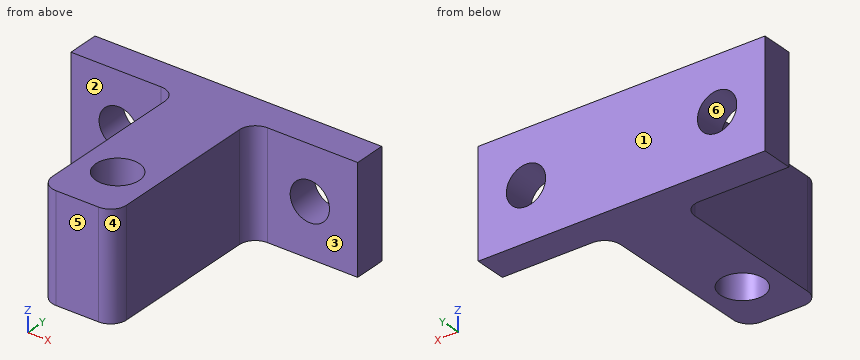
from build123d import *

# Parameters (mm, degrees)
SKETCH1_R           = 2.05
BOSS_EXTRUDE1_DEPTH = 5
FILLET1_R           = 1.5
SKETCH2_R           = 1.85
CUT_EXTRUDE1_DEPTH  = 21


with BuildPart() as part:
    # Sketch1 → Boss-Extrude1 (new body, symmetric)
    with BuildSketch(Plane.XY):
        Polygon((-13.502392344, 0), (-3.5, 0), (-3.5, -17), (3.5, -17), (3.5, 0), (13.502392344, 0), (13.502392344, 3), (-13.502392344, 3), align=None)
        with Locations((0, -12)):
            Circle(SKETCH1_R, mode=Mode.SUBTRACT)
    extrude(amount=BOSS_EXTRUDE1_DEPTH, both=True)

    # Fillet1
    fillet1_edges = [part.edges().sort_by_distance(p)[0] for p in [
        (3.5, 0, 0),
        (3.5, -17, 0),
        (-3.5, -17, 0),
        (-3.5, 0, 0),
    ]]
    fillet(fillet1_edges, radius=FILLET1_R)

    # Sketch2 → Cut-Extrude1 (cut, through all)
    with BuildSketch(Plane(origin=(0, 3, 0), x_dir=(1, 0, 0), z_dir=(0, 1, 0))):
        with Locations((-9, 0)):
            Circle(SKETCH2_R)
        with Locations((9, 0)):
            Circle(SKETCH2_R)
    extrude(amount=-CUT_EXTRUDE1_DEPTH, mode=Mode.SUBTRACT)


solid = part.part
Geometry check sheet. Reference: the model listing, model coordinates, mm. Face numbers are marked on the shaded views. A direction names the side the tool comes from. Coordinates: 2 decimals unless noted, no trailing zeros. Order: outer loops, then holes, each group sorted by start corner. A loop starts at its lowest first (then second) coordinate and runs counter-clockwise, first axis right, second up. Notation, with made-up numbers: (8, 82.25) - (20, 82.25) arc R23 ccw to (20, 110.25) - close; hole circle Ø5 at (84, 64.25). An arc over 180 degrees is marked (long way). Answer in a Markdown table with one row per item. Add a question column.
1) Set-up check for the marked faces 1, 2 and 3: record each of +Z, -Z, +X, -X, +Y, -Y from which the full face is reachable in a straight line by a thin tool's end or side.
2) Gauge pin test, flat ends, axial feed: P1, Ø3.5, axis at x = 0, y = -12, coming from the -Z side; P2, Ø3, axis at y = -0.5, z = -4, coming from the +X side; P3, Ø3, axis at y = -8.5, z = 2.5, coming from the -X side; P4, Ø5, axis at y = -9, z = 2.5, coming from the +X side. Record the tip position at first contact, or that the pin passes through.
3) Cross-section at A-A, the plane z = 0. Record the cut outline in (x, y).
4) Release check for a two-part mould opening along X. For the marked faces 4, 5 and 6 record: +X half, -X half, draft (parallel to the pull), parting line (faces both ways), or undercut.
5) Cross-section at D-D, the plane y = -13.5. Record the cut outline in (x, z).
6) Cross-section at B-B, the plane x = 9. Record the cut outline in (y, z).
7) Material ranges on line 1 along X through (y, z) = (1.5, 0); line 2 along Z through (x, y) = (9, 1); line 3 along Y through (x, z) = (0, 2.5), recorded low to high. Write a range as [from, to].
8) Cross-section at C-C, the plane z = -2.5. Record the cut outline in (x, y).
Check result:
| question | item | result |
|---|---|---|
| 1 | face 1 | +Z, -Z, +X, -X, +Y |
| 1 | face 2 | +Z, -Z, -X, -Y |
| 1 | face 3 | +Z, -Z, +X, -Y |
| 2 | P1 | passes through |
| 2 | P2 | stops at x = 13.5 |
| 2 | P3 | stops at x = -3.5 |
| 2 | P4 | stops at x = 3.5 |
| 3 | outline | (-13.5, 0) - (-10.85, 0) - (-10.85, 3) - (-13.5, 3) - close; (-7.15, 0) - (-5, 0) arc R1.5 cw to (-3.5, -1.5) - (-3.5, -15.5) arc R1.5 ccw to (-2, -17) - (2, -17) arc R1.5 ccw to (3.5, -15.5) - (3.5, -1.5) arc R1.5 cw to (5, 0) - (7.15, 0) - (7.15, 3) - (-7.15, 3) - close; (10.85, 0) - (13.5, 0) - (13.5, 3) - (10.85, 3) - close; hole circle Ø4.1 at (0, -12) |
| 4 | face 4 | +X half |
| 4 | face 5 | draft |
| 4 | face 6 | undercut |
| 5 | outline | (-3.5, -5) - (-1.4, -5) - (-1.4, 5) - (-3.5, 5) - close; (1.4, -5) - (3.5, -5) - (3.5, 5) - (1.4, 5) - close |
| 6 | outline | (0, -5) - (3, -5) - (3, -1.85) - (0, -1.85) - close; (0, 1.85) - (3, 1.85) - (3, 5) - (0, 5) - close |
| 7 | line 1 | x = [-13.5, -10.85], [-7.15, 7.15], [10.85, 13.5] |
| 7 | line 2 | z = [-5, -1.85], [1.85, 5] |
| 7 | line 3 | y = [-17, -14.05], [-9.95, 3] |
| 8 | outline | (-13.5, 0) - (-5, 0) arc R1.5 cw to (-3.5, -1.5) - (-3.5, -15.5) arc R1.5 ccw to (-2, -17) - (2, -17) arc R1.5 ccw to (3.5, -15.5) - (3.5, -1.5) arc R1.5 cw to (5, 0) - (13.5, 0) - (13.5, 3) - (-13.5, 3) - close; hole circle Ø4.1 at (0, -12) |
